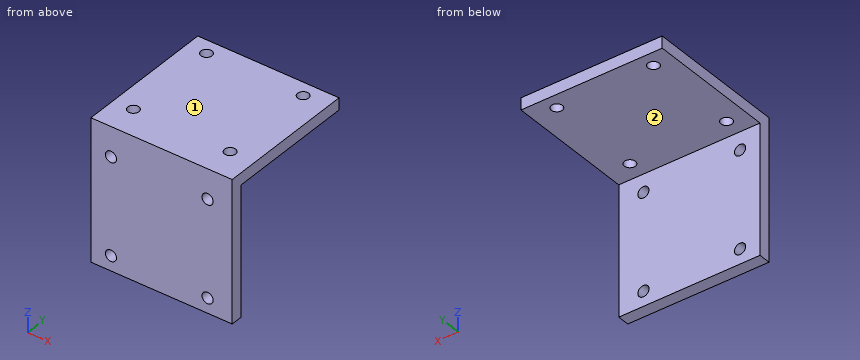
Autodesk Inventor part; units mm, degrees
ref_plane "YZ Plane" through (0, 0, 0) normal (1, 0, 0) x (0, 1, 0)
ref_plane "XZ Plane" through (0, 0, 0) normal (0, 1, 0) x (-1, 0, 0)
ref_plane "XY Plane" through (0, 0, 0) normal (0, 0, 1) x (1, 0, 0)
sketch "Sketch1" plane through (0, 0, 0) normal (1, 0, 0) x (0, 1, 0)
  line L0 (-7.48, 28.2623) -> (30.52, 28.2623)
  line L1 (30.52, 28.2623) -> (30.52, 25.0623)
  line L2 (30.52, 25.0623) -> (-4.28, 25.0623)
  line L3 (-4.28, 25.0623) -> (-4.28, -9.7377)
  line L4 (-4.28, -9.7377) -> (-7.48, -9.7377)
  line L5 (-7.48, -9.7377) -> (-7.48, 28.2623)
  dimension "d0" = 3.2
  dimension "d1" = 38
  dimension "d2" = 3.2
  dimension "d3" = 38
extrude "Extrusion1" add sketch "Sketch1" along normal blind 38
sketch "Sketch2" plane through (0, -7.48, -9.7377) normal (0, -1, 0) x (1, 0, 0)
  circle A0 centre (5.3744, 30) radius 1.5
  line L0 (0, 0) -> (0, 38)
  line L1 (0, 0) -> (38, 0)
  line L2 (38, 38) -> (38, 0)
  line L3 (0, 38) -> (38, 38)
  circle A1 centre (5.3744, 4) radius 1.5
  circle A2 centre (31.3744, 30) radius 1.5
  circle A3 centre (31.3744, 4) radius 1.5
  dimension "d13" = 26
  dimension "d16" = 26
  dimension "d19" = 8
  dimension "d20" = 3
extrude "Extrusion2" cut sketch "Sketch2" against normal up to next contours A0 | A1 | A2 | A3
sketch "Sketch3" plane through (0, -7.48, 28.2623) normal (0, 0, 1) x (1, 0, 0)
  circle A0 centre (5.3744, 34) radius 1.5
  line L0 (0, 0) -> (0, 38)
  line L1 (0, 0) -> (38, 0)
  line L2 (38, 38) -> (38, 0)
  line L3 (0, 38) -> (38, 38)
  circle A1 centre (5.3744, 8) radius 1.5
  circle A2 centre (31.3744, 34) radius 1.5
  circle A3 centre (31.3744, 8) radius 1.5
  point P0 (0, 7.48)
  dimension "d27" = 26
  dimension "d28" = 26
  dimension "d30" = 3
  dimension "d31" = 8
extrude "Extrusion3" cut sketch "Sketch3" against normal up to next contours A0 | A1 | A2 | A3
properties part number "Y_carriage_90_bearing_mount"
Verification items for the finished model (mm, model axes). Face numbers are marked on the shaded views. A direction names the side the tool comes from. Give positions to 0.01 mm unless a question says otherwise; leave off trailing zeros. Order: outer loops, then holes, each group sorted by start corner. A loop starts at its lowest first (then second) coordinate and runs counter-clockwise, first axis right, second up. Notation, with made-up numbers: M -2.75,62 L 21.25,62 A16 cw 21.25,82 Z; hole C -0.75,60.5 d6. An arc over 180 degrees is marked long. Answer as a JSON object with one key per item and string values. Group by question number.
1) Cross-section at D-D (y = 12.5). Enter the section's corners in (x, z).
2) Access from +Z, -Z, +X, -X, +Y, -Y to the whole of each face (thin tool, end or side, straight path). Record for the marked faces 1 and 2.
3) Cross-section at B-B (x = 6). Enter the section's corners in (y, z), then the cut area to 3 significant figures.
4) Cross-section at A-A (y = 0.52). Enter the section's corners in (x, z), then the cut area to 3 significant figures.
5) Depth check by flat-ended pin: pin 1 Ø2 at (y, z) = (-2, -5) entering from -X; pin 2 Ø17.5 at (x, z) = (26.5, 15) entering from +Y; pin 3 Ø10.5 at (x, y) = (25, 10) entering from -Z. Enter the tip coordinate at first touch or a pass-through.
6) Scan lines: line 1 along X through (y, z) = (-6, 19); line 2 along X through (y, z) = (0, 26); line 3 along Y through (x, z) = (18, -2). Record each from-to range of solid material in increasing order. Write a range as [from, to].
7) Cross-section at C-C (z = -5). Enter the section's corners in (x, y).
Result sheet:
{
 "1": {"outline": "M 0,25.06 L 38,25.06 L 38,28.26 L 0,28.26 Z"},
 "2": {"face 1": "+Z, +X, -X, +Y, -Y", "face 2": "-Z, +X, -X, +Y"},
 "3": {"outline": "M -7.48,-9.74 L -4.28,-9.74 L -4.28,-7.1 L -7.48,-7.1 Z; M -7.48,-4.37 L -4.28,-4.37 L -4.28,18.9 L -7.48,18.9 Z; M -7.48,21.63 L -4.28,21.63 L -4.28,25.06 L -0.84,25.06 L -0.84,28.26 L -7.48,28.26 Z; M 1.88,25.06 L 25.16,25.06 L 25.16,28.26 L 1.88,28.26 Z; M 27.88,25.06 L 30.52,25.06 L 30.52,28.26 L 27.88,28.26 Z", "area": "198 mm2"},
 "4": {"outline": "M 0,25.06 L 3.87,25.06 L 3.87,28.26 L 0,28.26 Z; M 6.87,25.06 L 29.87,25.06 L 29.87,28.26 L 6.87,28.26 Z; M 32.87,25.06 L 38,25.06 L 38,28.26 L 32.87,28.26 Z", "area": "102 mm2"},
 "5": {"pin 1": "passes through", "pin 2": "stops at y = -4.28", "pin 3": "stops at z = 25.06"},
 "6": {"line 1": "x = [0, 4.56], [6.18, 30.56], [32.18, 38]", "line 2": "x = [0, 3.97], [6.78, 29.97], [32.78, 38]", "line 3": "y = [-7.48, -4.28]"},
 "7": {"outline": "M 0,-7.48 L 4.07,-7.48 L 4.07,-4.28 L 0,-4.28 Z; M 6.68,-7.48 L 30.07,-7.48 L 30.07,-4.28 L 6.68,-4.28 Z; M 32.68,-7.48 L 38,-7.48 L 38,-4.28 L 32.68,-4.28 Z"}
}
